```python
from build123d import *

# Parameters (mm, degrees)
BOSS_EXTRUDE1_DEPTH = 5
SKETCH2_W           = 4.5
SKETCH2_H           = 55
CUT_EXTRUDE1_DEPTH  = 198.863589374
BOSS_EXTRUDE2_START = -5
SKETCH3_W           = 10
SKETCH3_H           = 30
BOSS_EXTRUDE2_DEPTH = 35
CHAMFER1_SIZE       = 2
SKETCH5_W           = 90
SKETCH5_H           = 5
BOSS_EXTRUDE3_DEPTH = 20
BOSS_EXTRUDE4_DEPTH = 5
BOSS_EXTRUDE5_DEPTH = 15
BOSS_EXTRUDE6_DEPTH = 20
BOSS_EXTRUDE7_DEPTH = 7
BOSS_EXTRUDE8_REACH = 248.625


with BuildPart() as part:
    # Sketch1 → Boss-Extrude1 (new body)
    with BuildSketch(Plane(origin=(0, 0, 0), x_dir=(1, 0, 0), z_dir=(0, 1, 0))):
        Polygon((-45, -30), (-45, -190), (45, -190), (45, -30), (55, -30), (55, 0), (-55, 0), (-55, -30), align=None)
    extrude(amount=BOSS_EXTRUDE1_DEPTH)

    # Sketch2 → Cut-Extrude1 (cut, through all)
    with BuildSketch(Plane(origin=(0, 5, 0), x_dir=(1, 0, 0), z_dir=(0, 1, 0))):
        with Locations((39.75, -112.5)):
            Rectangle(SKETCH2_W, SKETCH2_H)
        with Locations((-39.75, -112.5)):
            Rectangle(SKETCH2_W, SKETCH2_H)
    extrude(amount=-CUT_EXTRUDE1_DEPTH, mode=Mode.SUBTRACT)

    # Sketch3 → Boss-Extrude2 (add)
    with BuildSketch(Plane(origin=(0, 5, 0), x_dir=(1, 0, 0), z_dir=(0, 1, 0)).offset(BOSS_EXTRUDE2_START)):
        with Locations((50, -15)):
            Rectangle(SKETCH3_W, SKETCH3_H)
        with Locations((-50, -15)):
            Rectangle(SKETCH3_W, SKETCH3_H)
    extrude(amount=-BOSS_EXTRUDE2_DEPTH)

    # Chamfer1
    chamfer1_edges = [part.edges().sort_by_distance(p)[0] for p in [
        (-55, -15, 30),
        (-55, -15, 0),
        (55, -15, 0),
        (55, -15, 30),
        (45, -17.5, 30),
        (45, -17.5, 0),
        (-45, -17.5, 0),
        (-45, -17.5, 30),
    ]]
    chamfer(chamfer1_edges, length=CHAMFER1_SIZE)

    # Sketch5 → Boss-Extrude3 (add)
    with BuildSketch(Plane.XY.offset(190)):
        with Locations((0, 2.5)):
            Rectangle(SKETCH5_W, SKETCH5_H)
    extrude(amount=BOSS_EXTRUDE3_DEPTH)

    # Sketch8 → Boss-Extrude4 (add)
    with BuildSketch(Plane.ZY.offset(45)):
        Polygon((202.579910044, 0), (182.579910044, -63), (190, -63), (210, 0), align=None)
    boss_extrude4 = extrude(amount=-BOSS_EXTRUDE4_DEPTH)

    # Sketch9 → Boss-Extrude5 (add)
    with BuildSketch(Plane(origin=(-40, 0, 0), x_dir=(0, 0, -1), z_dir=(1, 0, 0))):
        Polygon((-190.952380952, -60), (-183.532290996, -60), (-182.579910044, -63), (-190, -63), align=None)
    boss_extrude5 = extrude(amount=BOSS_EXTRUDE5_DEPTH)

    # Sketch10 → Boss-Extrude6 (add)
    with BuildSketch(Plane.ZY.offset(45)):
        Polygon((190, -68), (190, -63), (190.952380952, -60), (192.452380952, -60), (191.5, -63), (191.5, -68), align=None)
    boss_extrude6 = extrude(amount=-BOSS_EXTRUDE6_DEPTH)

    # Mirror1: Boss-Extrude4, Boss-Extrude5, Boss-Extrude6 across plane
    add(boss_extrude4.mirror(Plane(origin=(0, 0, 0), x_dir=(0, 0, 1), z_dir=(1, 0, 0))))
    add(boss_extrude5.mirror(Plane(origin=(0, 0, 0), x_dir=(0, 0, 1), z_dir=(1, 0, 0))))
    add(boss_extrude6.mirror(Plane(origin=(0, 0, 0), x_dir=(0, 0, 1), z_dir=(1, 0, 0))))

    # Sketch11 → Boss-Extrude7 (add)
    with BuildSketch(Plane(origin=(0, 5, 0), x_dir=(1, 0, 0), z_dir=(0, 1, 0))):
        Polygon((45, -210), (45, -30), (53, -30), (55, -28), (55, -2), (53, 0), (-53, 0), (-55, -2), (-55, -28), (-53, -30), (-45, -30), (-45, -210), align=None)
        Polygon((51.757359313, -27), (42, -27), (42, -85), (42, -140), (42, -207), (-42, -207), (-42, -140), (-42, -85), (-42, -27), (-51.757359313, -27), (-52, -26.757359313), (-52, -3.242640687), (-51.757359313, -3), (51.757359313, -3), (52, -3.242640687), (52, -26.757359313), align=None, mode=Mode.SUBTRACT)
    extrude(amount=BOSS_EXTRUDE7_DEPTH)

    # Boss-Extrude8: up to this face of the body (flat: up to its plane)
    boss_extrude8_end = Plane(part.part.faces().sort_by_distance((45, -17.5, 15))[0])
    # Sketch12 → Boss-Extrude8 (add, up to the picked face)
    with BuildSketch(Plane(origin=(55, 0, 0), x_dir=(0, 0, -1), z_dir=(1, 0, 0)), mode=Mode.PRIVATE) as boss_extrude8_sk1:
        Polygon((0, -32), (12, -32), (12, -68), (2.5183809, -68), (2.5183809, -65), (9, -65), (9, -35), (0, -35), align=None)
    boss_extrude8_tool1 = split(extrude(boss_extrude8_sk1.sketch, amount=-BOSS_EXTRUDE8_REACH, mode=Mode.PRIVATE), bisect_by=boss_extrude8_end, keep=Keep.BOTH, mode=Mode.PRIVATE)
    add(boss_extrude8_tool1.solids().sort_by(Axis((55, -32.379473, -6), (-1, 0, 0)))[0])


solid = part.part
```
Read the model definition and answer for the solid it produces. Units are mm, in the model's axes. A direction names the side the tool comes from. Coordinates: 2 decimals unless noted, no trailing zeros. Order: outer loops, then holes, each group sorted by start corner. A loop starts at its lowest first (then second) coordinate and runs counter-clockwise, first axis right, second up. Notation, with made-up numbers: (34, -33.75) - (73, -33.75) arc R24 cw to (73, -11.75) - close; hole circle Ø11 at (-21.5, 67.5). An arc over 180 degrees is marked (long way). Answer as a JSON object with one key per item and string values. Group by question number.
Item 1: Flat-ended cylindrical pins translate along their axes: P1, Ø5.5, axis at x = -3.5, y = 9.5, coming from the -Z side; P2, Ø21, axis at y = -15.5, z = 196.5, coming from the -X side; P3, Ø1, axis at x = -1, z = 36.5, coming from the -Y side; P4, Ø23.5, axis at x = 20.5, y = -15, coming from the -Z side. Find the tip coordinate at first contact, or state that the pin passes through.
Item 2: Section C-C (z = 160) is taken. Give the vertices of the cut face in (x, y), plus the area to 3 significant figures.
Item 3: Section D-D (y = -24.5) is taken. Give the vertices of the cut face in (x, z).
Item 4: Section B-B (x = 31) is taken. Give the vertices of the cut face in (y, z), plus the area to 3 significant figures.
Item 5: The mould has two halves that part along X. Classify faces 1 (the face through (-55, -12, 15)), 2 (the face through (42.535, -30.42, 200.343)), 3 (the face through (-1, 8, 3)): +X half, -X half, draft (parallel to the pull), parting line (faces both ways), or undercut.
Item 6: Consider probe 1 along X at (y, z) = (-6, 26); probe 2 along Z at (x, y) = (40, 7.5); probe 3 along X at (y, z) = (6, 165.5). Determine where each line is inside the solid, lowest interval first. Write a range as from..to.
Item 7: A tool of negligible diameter and unlimited length cuts with its end or side. For faces 4 (the face through (45, 4, 134)), 5 (the face through (52, 8, 15)), 6 (the face through (-40, -30, 197)), from which of +Z, -Z, +X, -X, +Y, -Y can it reach the whole face along a straight path? Write none if from no direction.
Item 8: Section A-A (z = 103.5) is taken. Give the vertices of the cut face in (x, y).
Results are:
{
 "1": {"P1": "stops at z = 0", "P2": "stops at x = -45", "P3": "stops at y = 0", "P4": "passes through"},
 "2": {"outline": "(-45, 0) - (45, 0) - (45, 12) - (42, 12) - (42, 5) - (-42, 5) - (-42, 12) - (-45, 12) - close", "area": "492 mm^2"},
 "3": {"outline": "(-55, 2) - (-53, 0) - (-47, 0) - (-45, 2) - (-45, 28) - (-47, 30) - (-53, 30) - (-55, 28) - close; (-45, 194.8) - (-40, 194.8) - (-40, 202.22) - (-45, 202.22) - close; (40, 194.8) - (45, 194.8) - (45, 202.22) - (40, 202.22) - close; (45, 2) - (47, 0) - (53, 0) - (55, 2) - (55, 28) - (53, 30) - (47, 30) - (45, 28) - close"},
 "4": {"outline": "(-68, 190) - (-63, 190) - (-63, 182.58) - (-60, 183.53) - (-60, 192.45) - (-63, 191.5) - (-68, 191.5) - close; (0, 0) - (12, 0) - (12, 3) - (5, 3) - (5, 207) - (12, 207) - (12, 210) - (0, 210) - close", "area": "1,130 mm^2"},
 "5": {"face 1": "-X half", "face 2": "draft", "face 3": "undercut"},
 "6": {"probe 1": "x = -55..-45, 45..55", "probe 2": "z = 0..3, 207..210", "probe 3": "x = -45..-42, 42..45"},
 "7": {"face 4": "+Z, +X, +Y, -Y", "face 5": "+Y", "face 6": "+Z, -Z"},
 "8": {"outline": "(-45, 0) - (-42, 0) - (-42, 12) - (-45, 12) - close; (-37.5, 0) - (37.5, 0) - (37.5, 5) - (-37.5, 5) - close; (42, 0) - (45, 0) - (45, 12) - (42, 12) - close"}
}
